Design review of the part built by this model. Coordinates are the model's own, in mm. A direction names the side the tool comes from. Coordinates: 2 decimals unless noted, no trailing zeros. Loops run counter-clockwise (first coordinate to the right, second up) from the corner with the lowest first, then second, coordinate; pieces in that order, holes last. Notation, with made-up numbers: (-33.5, -35.5) -> (11.5, -35.5) arc R22 cw to (11.5, 2.5) -> close; hole circle Ø6 at (50.5, -20.5). An arc over 180 degrees is marked (long way). Answer as a JSON object with one key per item and string values.
```python
from build123d import *

# Parameters (mm, degrees)
BOSS_EXTRUDE1_DEPTH  = 15
SKETCH2_W            = 12
SKETCH2_H            = 10
BOSS_EXTRUDE2_DEPTH  = 1
FILLET1_R            = 1
SKETCH3_R            = 1
BOSS_EXTRUDE3_DEPTH  = 2
SKETCH4_R            = 1.5
BOSS_EXTRUDE4_DEPTH  = 2.5
SKETCH12_R           = 2.5
BOSS_EXTRUDE11_DEPTH = 1
SKETCH13_R           = 1.5
CUT_EXTRUDE4_DEPTH   = 0.5
FILLET5_R            = 0.6
SKETCH15_W           = 1
SKETCH15_H           = 2
CUT_EXTRUDE5_DEPTH   = 2
CUT_EXTRUDE6_DEPTH   = 0.2
CUT_EXTRUDE7_START   = -0.2
CUT_EXTRUDE7_DEPTH   = 0.2
SKETCH31_W           = 0.5
SKETCH31_H           = 2
BOSS_EXTRUDE16_DEPTH = 2
FILLET9_R            = 0.6
SKETCH32_R           = 0.5
CUT_EXTRUDE10_DEPTH  = 2
CUT_EXTRUDE11_START  = -2
SKETCH33_R           = 0.5
CUT_EXTRUDE11_DEPTH  = 2
BOSS_EXTRUDE17_DEPTH = 1
FILLET10_R           = 1
SKETCH34_R           = 1.5
BOSS_EXTRUDE18_DEPTH = 4
SKETCH35_W           = 12
SKETCH35_H           = 10
BOSS_EXTRUDE19_DEPTH = 1
SKETCH36_R           = 2
BOSS_EXTRUDE20_DEPTH = 1
CUT_EXTRUDE12_START  = -2
SKETCH37_R           = 1.5
CUT_EXTRUDE12_DEPTH  = 2
FILLET11_R           = 1
SKETCH38_R           = 0.5
CUT_EXTRUDE13_DEPTH  = 2
SKETCH39_R           = 0.75
CUT_EXTRUDE14_DEPTH  = 9.3
CHAMFER1_SIZE        = 0.3
SKETCH40_R           = 0.5
CUT_EXTRUDE15_DEPTH  = 1
SKETCH41_R           = 0.5
CUT_EXTRUDE16_DEPTH  = 1
SKETCH42_R           = 0.5
CUT_EXTRUDE17_DEPTH  = 1
SKETCH43_R           = 0.5
CUT_EXTRUDE18_DEPTH  = 1


with BuildPart() as part:
    # Sketch1 → Boss-Extrude1 (new body)
    with BuildSketch(Plane.XY):
        with BuildLine():
            Line((-6, -1.25), (-6, 1.25))
            ThreePointArc((-6, 1.25), (-5.317704321, 3.503469547), (-3.5, 5))
            Line((-3.5, 5), (3.5, 5))
            ThreePointArc((3.5, 5), (5.317704321, 3.503469547), (6, 1.25))
            Line((6, 1.25), (6, -1.25))
            ThreePointArc((6, -1.25), (5.317704321, -3.503469547), (3.5, -5))
            Line((3.5, -5), (-3.5, -5))
            ThreePointArc((-3.5, -5), (-5.317704321, -3.503469547), (-6, -1.25))
        make_face()
    extrude(amount=-BOSS_EXTRUDE1_DEPTH)

    # Sketch2 → Boss-Extrude2 (add)
    with BuildSketch(Plane(origin=(0, 0, -15), x_dir=(-1, 0, 0), z_dir=(0, 0, -1))):
        Rectangle(SKETCH2_W, SKETCH2_H)
    extrude(amount=BOSS_EXTRUDE2_DEPTH)

    # Fillet1
    fillet1_edges = [part.edges().sort_by_distance(p)[0] for p in [
        (6, 5, -15.5),
        (6, -5, -15.5),
        (-6, -5, -15.5),
        (-6, 5, -15.5),
    ]]
    fillet(fillet1_edges, radius=FILLET1_R)

    # Sketch3 → Boss-Extrude3 (add)
    with BuildSketch(Plane(origin=(0, 0, -16), x_dir=(-1, 0, 0), z_dir=(0, 0, -1))):
        Circle(SKETCH3_R)
    extrude(amount=BOSS_EXTRUDE3_DEPTH)

    # Sketch4 → Boss-Extrude4 (add)
    with BuildSketch(Plane(origin=(0, 0, -16), x_dir=(-1, 0, 0), z_dir=(0, 0, -1))):
        with Locations((4.3, 3.3)):
            Circle(SKETCH4_R)
        with Locations((-4.3, -3.3)):
            Circle(SKETCH4_R)
    extrude(amount=BOSS_EXTRUDE4_DEPTH)

    # Sketch12 → Boss-Extrude11 (add)
    with BuildSketch(Plane.XY):
        Circle(SKETCH12_R)
    extrude(amount=BOSS_EXTRUDE11_DEPTH)

    # Sketch13 → Cut-Extrude4 (cut)
    with BuildSketch(Plane.XY.offset(1)):
        Circle(SKETCH13_R)
    extrude(amount=-CUT_EXTRUDE4_DEPTH, mode=Mode.SUBTRACT)

    # Fillet5
    fillet5_edges = [part.edges().sort_by_distance(p)[0] for p in [
        (-2.5, 0, 1),
    ]]
    fillet(fillet5_edges, radius=FILLET5_R)

    # Sketch15 → Cut-Extrude5 (cut)
    with BuildSketch(Plane.XY):
        with Locations((-5.5, 0)):
            Rectangle(SKETCH15_W, SKETCH15_H)
        with Locations((5.5, 0)):
            Rectangle(SKETCH15_W, SKETCH15_H)
    extrude(amount=-CUT_EXTRUDE5_DEPTH, mode=Mode.SUBTRACT)

    # Sketch22 → Cut-Extrude6 (cut)
    with BuildSketch(Plane(origin=(0, 5, 0), x_dir=(1, 0, 0), z_dir=(0, 1, 0))):
        with BuildLine():
            Line((-2.4, 8.5), (-2.4, 13.5))
            ThreePointArc((-2.4, 13.5), (-2.1, 13.8), (-1.8, 13.5))
            Line((-1.8, 13.5), (-1.8, 8.5))
            ThreePointArc((-1.8, 8.5), (-2.1, 8.2), (-2.4, 8.5))
        make_face()
        with BuildLine():
            Line((2.2, 8.5), (2.2, 13.5))
            ThreePointArc((2.2, 13.5), (2.5, 13.8), (2.8, 13.5))
            Line((2.8, 13.5), (2.8, 8.5))
            ThreePointArc((2.8, 8.5), (2.5, 8.2), (2.2, 8.5))
        make_face()
    extrude(amount=-CUT_EXTRUDE6_DEPTH, mode=Mode.SUBTRACT)

    # Sketch23 → Cut-Extrude7 (cut)
    with BuildSketch(Plane.XZ.offset(5).offset(CUT_EXTRUDE7_START)):
        with BuildLine():
            Line((-2.8, -13.5), (-2.8, -8.5))
            ThreePointArc((-2.8, -8.5), (-2.5, -8.2), (-2.2, -8.5))
            Line((-2.2, -8.5), (-2.2, -13.5))
            ThreePointArc((-2.2, -13.5), (-2.5, -13.8), (-2.8, -13.5))
        make_face()
        with BuildLine():
            Line((2.2, -13.5), (2.2, -8.5))
            ThreePointArc((2.2, -8.5), (2.5, -8.2), (2.8, -8.5))
            Line((2.8, -8.5), (2.8, -13.5))
            ThreePointArc((2.8, -13.5), (2.5, -13.8), (2.2, -13.5))
        make_face()
    extrude(amount=CUT_EXTRUDE7_DEPTH, mode=Mode.SUBTRACT)

    # Sketch31 → Boss-Extrude16 (add)
    with BuildSketch(Plane.XY):
        with Locations((-4.55, -0.008606945)):
            Rectangle(SKETCH31_W, SKETCH31_H)
        with Locations((4.55, -0.039338836)):
            Rectangle(SKETCH31_W, SKETCH31_H)
    extrude(amount=BOSS_EXTRUDE16_DEPTH)

    # Fillet9
    fillet9_edges = [part.edges().sort_by_distance(p)[0] for p in [
        (-4.55, -1.008606945, 2),
        (-4.55, 0.991393055, 2),
        (4.55, 0.960661164, 2),
        (4.55, -1.039338836, 2),
    ]]
    fillet(fillet9_edges, radius=FILLET9_R)

    # Sketch32 → Cut-Extrude10 (cut)
    with BuildSketch(Plane.ZY.offset(4.8)):
        with Locations((1.35, 0)):
            Circle(SKETCH32_R)
    extrude(amount=-CUT_EXTRUDE10_DEPTH, mode=Mode.SUBTRACT)

    # Sketch33 → Cut-Extrude11 (cut)
    with BuildSketch(Plane(origin=(4.8, 0, 0), x_dir=(0, 0, -1), z_dir=(1, 0, 0)).offset(CUT_EXTRUDE11_START)):
        with Locations(Location((-1.35, 0, 0), (0, 0, 180))):
            Circle(SKETCH33_R)
    extrude(amount=CUT_EXTRUDE11_DEPTH, mode=Mode.SUBTRACT)

    # Sketch24 → Boss-Extrude17 (add)
    with BuildSketch(Plane(origin=(0, 0, -18.5), x_dir=(-1, 0, 0), z_dir=(0, 0, -1))):
        Polygon((2, -5), (2, 1.11), (6, 1.11), (6, 5), (-6, 5), (-6, -5), align=None)
    extrude(amount=BOSS_EXTRUDE17_DEPTH)

    # Fillet10
    fillet10_edges = [part.edges().sort_by_distance(p)[0] for p in [
        (6, 5, -19),
        (6, -5, -19),
        (-2, -5, -19),
        (-6, 5, -19),
    ]]
    fillet(fillet10_edges, radius=FILLET10_R)

    # Sketch34 → Boss-Extrude18 (add)
    with BuildSketch(Plane(origin=(0, 0, -19.5), x_dir=(-1, 0, 0), z_dir=(0, 0, -1))):
        with Locations((-4.3, -3.3)):
            Circle(SKETCH34_R)
        with Locations((4.3, 3.3)):
            Circle(SKETCH34_R)
    extrude(amount=BOSS_EXTRUDE18_DEPTH)

    # Sketch35 → Boss-Extrude19 (add)
    with BuildSketch(Plane(origin=(0, 0, -23.5), x_dir=(-1, 0, 0), z_dir=(0, 0, -1))):
        Rectangle(SKETCH35_W, SKETCH35_H)
    extrude(amount=BOSS_EXTRUDE19_DEPTH)

    # Sketch36 → Boss-Extrude20 (add)
    with BuildSketch(Plane(origin=(0, 0, -24.5), x_dir=(-1, 0, 0), z_dir=(0, 0, -1))):
        Circle(SKETCH36_R)
    extrude(amount=BOSS_EXTRUDE20_DEPTH)

    # Sketch37 → Cut-Extrude12 (cut)
    with BuildSketch(Plane(origin=(0, 0, -25.5), x_dir=(-1, 0, 0), z_dir=(0, 0, -1)).offset(CUT_EXTRUDE12_START)):
        with Locations(Location((0, 0, 0), (0, 0, 180))):
            Circle(SKETCH37_R)
    extrude(amount=CUT_EXTRUDE12_DEPTH, mode=Mode.SUBTRACT)

    # Fillet11
    fillet11_edges = [part.edges().sort_by_distance(p)[0] for p in [
        (6, 5, -24),
        (6, -5, -24),
        (-6, -5, -24),
        (-6, 5, -24),
    ]]
    fillet(fillet11_edges, radius=FILLET11_R)

    # Sketch38 → Cut-Extrude13 (cut)
    with BuildSketch(Plane(origin=(0, 0, -24.5), x_dir=(-1, 0, 0), z_dir=(0, 0, -1))):
        with Locations((-4.5, 0)):
            Circle(SKETCH38_R)
        with Locations((4.5, 0)):
            Circle(SKETCH38_R)
    extrude(amount=-CUT_EXTRUDE13_DEPTH, mode=Mode.SUBTRACT)

    # Sketch39 → Cut-Extrude14 (cut)
    with BuildSketch(Plane(origin=(0, 0, -24.5), x_dir=(-1, 0, 0), z_dir=(0, 0, -1))):
        with Locations((-4.3, -3.3)):
            Circle(SKETCH39_R)
        with Locations((4.3, 3.3)):
            Circle(SKETCH39_R)
    extrude(amount=-CUT_EXTRUDE14_DEPTH, mode=Mode.SUBTRACT)

    # Chamfer1
    chamfer1_edges = [part.edges().sort_by_distance(p)[0] for p in [
        (5.05, -3.3, -24.5),
        (-3.55, 3.3, -24.5),
    ]]
    chamfer(chamfer1_edges, length=CHAMFER1_SIZE)

    # Sketch40 → Cut-Extrude15 (cut)
    with BuildSketch(Plane(origin=(0, 0, -19.5), x_dir=(-1, 0, 0), z_dir=(0, 0, -1))):
        Circle(SKETCH40_R)
    extrude(amount=-CUT_EXTRUDE15_DEPTH, mode=Mode.SUBTRACT)

    # Sketch41 → Cut-Extrude16 (cut)
    with BuildSketch(Plane(origin=(0, 0, -24.5), x_dir=(-1, 0, 0), z_dir=(0, 0, -1))):
        with Locations((3.22, -1.25)):
            Circle(SKETCH41_R)
        with Locations((-3.22, 1.25)):
            Circle(SKETCH41_R)
    extrude(amount=-CUT_EXTRUDE16_DEPTH, mode=Mode.SUBTRACT)

    # Sketch42 → Cut-Extrude17 (cut)
    with BuildSketch(Plane(origin=(0, 0, -19.5), x_dir=(-1, 0, 0), z_dir=(0, 0, -1))):
        with Locations((-3.22, 1.25)):
            Circle(SKETCH42_R)
    extrude(amount=-CUT_EXTRUDE17_DEPTH, mode=Mode.SUBTRACT)

    # Sketch43 → Cut-Extrude18 (cut)
    with BuildSketch(Plane(origin=(0, 0, -16), x_dir=(-1, 0, 0), z_dir=(0, 0, -1))):
        with Locations((3.22, -1.25)):
            Circle(SKETCH43_R)
    extrude(amount=-CUT_EXTRUDE18_DEPTH, mode=Mode.SUBTRACT)


solid = part.part
```
1) Wall thickness on probe 1 along Z at (x, y) = (0.5, -3.5); probe 2 along Z at (x, y) = (1, 1.25); probe 3 along Y at (x, z) = (-4.3, -20.25): over which ranges is each line inside the solid? List them lowest first.
Completed:
{"probe 1": "-24.5 to -23.5, -19.5 to -18.5, -16 to 0", "probe 2": "-25.5 to -23.5, -19.5 to -18.5, -16 to 1", "probe 3": "1.8 to 2.55, 4.05 to 4.8"}
2) The part is to be moulded in two halves that separate along Z. For faces 1 (the cylindrical face through (-3.19, 4.31, -17.23)), 2 (the cylindrical face through (-0.54, -2.44, 0.2)), 3 (the flat face through (-5.5, 0, -2)), say which applies: pulls with the +Z half, pulls with the -Z half, needs draft (parallel to the pull), parting line crosses it, or undercut.
Completed:
{"face 1": "undercut", "face 2": "needs draft", "face 3": "pulls with the +Z half"}
3) Clearance check with flat-ended pins moving along their axes: pin 1 Ø1.1 at (x, z) = (-5.5, -1) entering from +Y; pin 2 Ø0.5 at (x, y) = (-3.5, -1.5) entering from -Z; pin 3 Ø1.1 at (x, y) = (0.5, 1) entering from +Z. State where each tip first meets the part, or that it passes through.
Completed:
{"pin 1": "y = 3.98", "pin 2": "z = -24.5", "pin 3": "z = 1"}
4) For faces 4 (the flat face through (5.5, 1, -1)), 5 (the flat face through (4, -3, -15.2)), 6 (the flat face through (-5.5, 1, -1)), 7 (the cylindrical face through (5.336, -3.476, -7.395)), list the 3-axis set-ups (+Z, -Z, +X, -X, +Y, -Y) from which the entire face can be reached by the end or side of a thin tool; tool diameter is ignored.
Completed:
{"face 4": "+Z, +X", "face 5": "-Z", "face 6": "+Z, -X", "face 7": "+Z, +X, -Y"}
5) Add section A-A, the plane z = -22. Give the boundary of the cut face in (x, y).
Completed:
{"outline": "circle Ø3 at (-4.3, 3.3); circle Ø3 at (4.3, -3.3); hole circle Ø1.5 at (-4.3, 3.3); hole circle Ø1.5 at (4.3, -3.3)"}
